The listing builds one solid part. Answer for the finished solid, in the listing's coordinates (mm). Face numbers are marked on the shaded views. A direction names the side the tool comes from. Coordinates: 2 decimals unless noted, no trailing zeros. Order: outer loops, then holes, each group sorted by start corner. A loop starts at its lowest first (then second) coordinate and runs counter-clockwise, first axis right, second up. Notation, with made-up numbers: (-35, 58.25) - (21, 58.25) arc R8 cw to (21, 68.25) - close; hole circle Ø9 at (74.25, -5.5). An arc over 180 degrees is marked (long way). Use a Markdown table: item, result. Add a question column.
Item 1: Flat-ended cylindrical pins translate along their axes: P1, Ø0.8, axis at x = 71, y = 11, coming from the -Z side; P2, Ø1, axis at x = 7, y = 24, coming from the -Z side; P3, Ø7, axis at y = 10.5, z = 10, coming from the +X side. Find the tip coordinate at first contact, or state that the pin passes through.
Item 2: For the marked faces 1 and 2, determine the directions among +Z, -Z, +X, -X, +Y, -Y from which every point of the face is accessible in a straight line to the end or side of a thin tool.
Item 3: The part is cut by section C-C, the plane z = 11. Give the vertices of the cut face in (x, y), then the cut area to 3 significant figures.
Item 4: The mould has two halves that part along X. Classify the marked faces 3, 4 and 5: released by +X, released by -X, zero draft, split by the parting line, or undercut.
Item 5: The part is cut by section B-B, the plane x = 30. Give the vertices of the cut face in (y, z).
Item 6: Find the intervals of material crossed by line 1 along X through (y, z) = (18, 14); line 2 along Y through (x, z) = (36, 13.75); line 3 along Y through (x, z) = (35, 14.75), in increasing order.
Item 7: The part is cut by section A-A, the plane y = 23. Give the vertices of the cut face in (x, z), then the cut area to 3 significant figures.
Item 8: The part is cut by section D-D, the plane x = 5. Give the vertices of the cut face in (y, z), then the cut area to 3 significant figures.
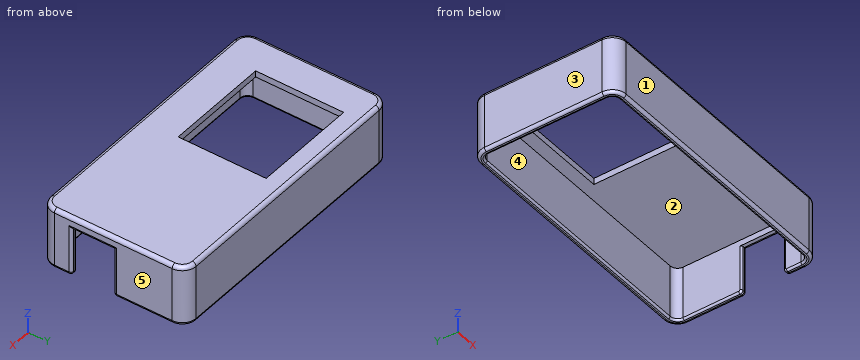
from build123d import *

# Parameters (mm, degrees)
BOSS_EXTRU_1_DEPTH      = 14.6
COQUE1_T                = 1.7
ESQUISSE7_W             = 1.7
ESQUISSE7_H             = 11.355170452
ENL_V_MAT_EXTRU_2_DEPTH = 13
CONG_2_R                = 0.75
ESQUISSE9_W             = 28.120859144
ESQUISSE9_H             = 23.752570345
ENL_V_MAT_EXTRU_3_DEPTH = 3
CONG_4_R                = 1
CONG_5_R                = 0.75
CONG_6_R                = 0.5


with BuildPart() as part:
    # Esquisse1 → Boss.-Extru.1 (new body)
    with BuildSketch(Plane.XY):
        with BuildLine():
            Line((2, 0), (68.4, 0))
            ThreePointArc((68.4, 0), (69.814213562, 0.585786438), (70.4, 2))
            Line((70.4, 2), (70.4, 33.8))
            ThreePointArc((70.4, 33.8), (69.814213562, 35.214213562), (68.4, 35.8))
            Line((68.4, 35.8), (2, 35.8))
            ThreePointArc((2, 35.8), (0.585786438, 35.214213562), (0, 33.8))
            Line((0, 33.8), (0, 2))
            ThreePointArc((0, 2), (0.585786438, 0.585786438), (2, 0))
        make_face()
    extrude(amount=BOSS_EXTRU_1_DEPTH)

    # Coque1
    coque1_openings = [part.faces().sort_by_distance(p)[0] for p in [
        (35.2, 17.9, 0),
    ]]
    offset(amount=COQUE1_T, openings=coque1_openings, kind=Kind.INTERSECTION)

    # Esquisse7 → Enlèv. mat.-Extru.2 (cut)
    with BuildSketch(Plane(origin=(0, 0, 0), x_dir=(-1, 0, 0), z_dir=(0, 0, -1))):
        with Locations((-71.25, 12.322414774)):
            Rectangle(ESQUISSE7_W, ESQUISSE7_H)
    extrude(amount=-ENL_V_MAT_EXTRU_2_DEPTH, mode=Mode.SUBTRACT)

    # Congé2
    cong_2_edges = [part.edges().sort_by_distance(p)[0] for p in [
        (71.25, 6.644829548, 0),
        (71.25, 18, 0),
    ]]
    fillet(cong_2_edges, radius=CONG_2_R)

    # Esquisse9 → Enlèv. mat.-Extru.3 (cut)
    with BuildSketch(Plane.XY.offset(16.3)):
        with Locations((22.126551481, 20.566590434)):
            Rectangle(ESQUISSE9_W, ESQUISSE9_H)
    extrude(amount=-ENL_V_MAT_EXTRU_3_DEPTH, mode=Mode.SUBTRACT)

    # Congé4
    cong_4_edges = [part.edges().sort_by_distance(p)[0] for p in [
        (-0.61629509, -0.61629509, 16.3),
        (35.2, -1.7, 16.3),
        (71.01629509, -0.61629509, 16.3),
        (72.1, 17.9, 16.3),
        (71.01629509, 36.41629509, 16.3),
        (35.2, 37.5, 16.3),
        (-0.61629509, 36.41629509, 16.3),
        (-1.7, 17.9, 16.3),
    ]]
    fillet(cong_4_edges, radius=CONG_4_R)

    # Congé5
    cong_5_edges = [part.edges().sort_by_distance(p)[0] for p in [
        (-1.7, 17.9, 0),
        (-0.61629509, 36.41629509, 0),
        (72.1, 12.322414774, 13),
        (72.1, 6.644829548, 6.875),
        (72.1, 18, 6.875),
        (72.1, 26.275, 0),
        (72.1, 18.219669914, 0.219669914),
        (72.1, 6.425159634, 0.219669914),
        (35.2, 37.5, 0),
        (71.01629509, 36.41629509, 0),
        (72.1, 3.947414774, 0),
        (71.01629509, -0.61629509, 0),
        (35.2, -1.7, 0),
        (-0.61629509, -0.61629509, 0),
    ]]
    fillet(cong_5_edges, radius=CONG_5_R)

    # Congé6
    cong_6_edges = [part.edges().sort_by_distance(p)[0] for p in [
        (0.585786438, 35.214213562, 0),
        (0, 17.9, 0),
        (0.585786438, 0.585786438, 0),
        (35.2, 0, 0),
        (69.814213562, 0.585786438, 0),
        (70.4, 3.947414774, 0),
        (69.814213562, 35.214213562, 0),
        (35.2, 35.8, 0),
        (70.4, 18, 6.875),
        (70.4, 6.644829548, 6.875),
        (70.4, 26.275, 0),
        (70.4, 18.219669914, 0.219669914),
        (70.4, 6.425159634, 0.219669914),
    ]]
    fillet(cong_6_edges, radius=CONG_6_R)


solid = part.part
Solution:
| question | item | result |
|---|---|---|
| 1 | P1 | stops at z = 13 |
| 1 | P2 | stops at z = 14.6 |
| 1 | P3 | stops at x = 72.06 |
| 2 | face 1 | +Z, -Z, +X, -X, -Y |
| 2 | face 2 | -Z |
| 3 | outline | (-1.7, 2) arc R3.7 ccw to (2, -1.7) - (68.4, -1.7) arc R3.7 ccw to (72.1, 2) - (72.1, 5.89) arc R0.75 ccw to (71.35, 6.64) - (70.9, 6.64) arc R0.5 ccw to (70.4, 6.14) - (70.4, 2) arc R2 cw to (68.4, 0) - (2, 0) arc R2 cw to (0, 2) - (0, 33.8) arc R2 cw to (2, 35.8) - (68.4, 35.8) arc R2 cw to (70.4, 33.8) - (70.4, 18.5) arc R0.5 ccw to (70.9, 18) - (71.35, 18) arc R0.75 ccw to (72.1, 18.75) - (72.1, 33.8) arc R3.7 ccw to (68.4, 37.5) - (2, 37.5) arc R3.7 ccw to (-1.7, 33.8) - close |
| 3 | area | 345 mm2 |
| 4 | face 3 | released by -X |
| 4 | face 4 | undercut |
| 4 | face 5 | released by +X |
| 5 | outline | (-1.7, 0.75) arc R0.75 ccw to (-0.95, 0) - (-0.5, 0) arc R0.5 ccw to (0, 0.5) - (0, 14.6) - (8.69, 14.6) - (8.69, 16.3) - (-0.7, 16.3) arc R1 ccw to (-1.7, 15.3) - close; (32.44, 14.6) - (35.8, 14.6) - (35.8, 0.5) arc R0.5 ccw to (36.3, 0) - (36.75, 0) arc R0.75 ccw to (37.5, 0.75) - (37.5, 15.3) arc R1 ccw to (36.5, 16.3) - (32.44, 16.3) - close |
| 6 | line 1 | x = -1.7 to 0, 70.4 to 72.1 |
| 6 | line 2 | y = -1.7 to 0, 35.8 to 37.5 |
| 6 | line 3 | y = -1.7 to 8.69, 32.44 to 37.5 |
| 7 | outline | (-1.7, 0.75) arc R0.75 ccw to (-0.95, 0) - (-0.5, 0) arc R0.5 ccw to (0, 0.5) - (0, 14.6) - (8.07, 14.6) - (8.07, 16.3) - (-0.7, 16.3) arc R1 ccw to (-1.7, 15.3) - close; (36.19, 14.6) - (70.4, 14.6) - (70.4, 0.5) arc R0.5 ccw to (70.9, 0) - (71.35, 0) arc R0.75 ccw to (72.1, 0.75) - (72.1, 15.3) arc R1 ccw to (71.1, 16.3) - (36.19, 16.3) - close |
| 7 | area | 127 mm2 |
| 8 | outline | (-1.7, 0.75) arc R0.75 ccw to (-0.95, 0) - (-0.5, 0) arc R0.5 ccw to (0, 0.5) - (0, 14.6) - (35.8, 14.6) - (35.8, 0.5) arc R0.5 ccw to (36.3, 0) - (36.75, 0) arc R0.75 ccw to (37.5, 0.75) - (37.5, 15.3) arc R1 ccw to (36.5, 16.3) - (-0.7, 16.3) arc R1 ccw to (-1.7, 15.3) - close |
| 8 | area | 116 mm2 |
